Geometry check sheet. Reference: drawing and pictorial views, mm from the part's lowest x, y, z. A direction names the side the tool comes from. Round coordinates to 2 decimals unless told otherwise and drop trailing zeros. Write each loop counter-clockwise with the first axis right and the second up, starting at its lowest first coordinate (ties: lowest second). Pieces come first, ordered by that corner, then holes. Notation, with made-up numbers: M -23.5,47 L 4.5,47 A31 ccw 4.5,74 Z; hole C 75.25,85.5 d6. An arc over 180 degrees is marked long. One line per item, written item: value. Start each with the question number.
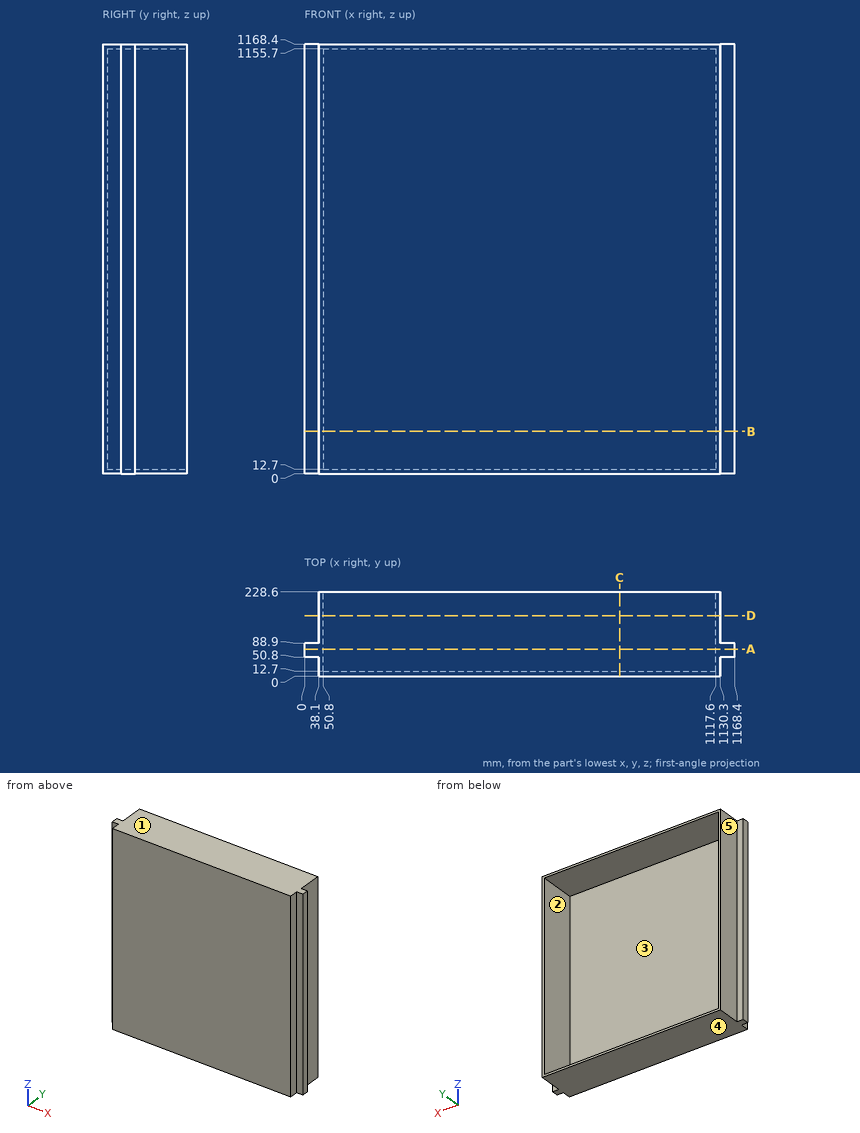
1) Access from +Z, -Z, +X, -X, +Y, -Y to the whole of each face (thin tool, end or side, straight path). Record for the marked faces 1 and 2.
2) Gauge pin test, flat ends, axial feed: pin 1 Ø19 at (x, z) = (1140.5, 494.5) entering from -Y; pin 2 Ø10 at (x, z) = (166, 423.5) entering from +Y; pin 3 Ø2 at (y, z) = (147.5, 708) entering from -X. Record the tip position at first contact, or that the pin passes through.
3) Cross-section at D-D (y = 164). Record the boundary of the cut face in (x, z), then the cut area to 3 significant figures.
4) Thickness scan on line 1 (Z direction, x = 68, y = 71); line 2 (X direction, y = 132, z = 960); line 3 (X direction, y = 84, z = 931.5). Record the ranges inside material, lowest first.
5) Mould release check, pull along X, two halves, no side actions. Record for the marked faces 3, 4 and 5: pulls with the +X half, pulls with the -X half, needs draft (parallel to the pull), parting line crosses it, or undercut.
6) Cross-section at A-A (y = 73). Record the boundary of the cut face in (x, z), then the cut area to 3 significant figures.
7) Cross-section at B-B (z = 115.5). Record the boundary of the cut face in (x, y), then the cut area to 3 significant figures.
8) Cross-section at C-C (x = 856). Record the boundary of the cut face in (y, z).
Results below:
1. face 1: +Z, +X, -X, +Y, -Y
1. face 2: +Y
2. pin 1: stops at y = 50.8
2. pin 2: stops at y = 12.7
2. pin 3: stops at x = 38.1
3. outline: M 38.1,0 L 1130.3,0 L 1130.3,1168.4 L 38.1,1168.4 Z; hole M 50.8,12.7 L 1117.6,12.7 L 1117.6,1155.7 L 50.8,1155.7 Z
3. area: 56,800 mm²
4. line 1: z = 0 to 12.7, 1155.7 to 1168.4
4. line 2: x = 38.1 to 50.8, 1117.6 to 1130.3
4. line 3: x = 0 to 50.8, 1117.6 to 1168.4
5. face 3: undercut
5. face 4: needs draft
5. face 5: pulls with the -X half
6. outline: M 0,0 L 1168.4,0 L 1168.4,1168.4 L 0,1168.4 Z; hole M 50.8,12.7 L 1117.6,12.7 L 1117.6,1155.7 L 50.8,1155.7 Z
6. area: 146,000 mm²
7. outline: M 0,50.8 L 38.1,50.8 L 38.1,0 L 1130.3,0 L 1130.3,50.8 L 1168.4,50.8 L 1168.4,88.9 L 1130.3,88.9 L 1130.3,228.6 L 1117.6,228.6 L 1117.6,12.7 L 50.8,12.7 L 50.8,228.6 L 38.1,228.6 L 38.1,88.9 L 0,88.9 Z
7. area: 22,300 mm²
8. outline: M 0,0 L 228.6,0 L 228.6,12.7 L 12.7,12.7 L 12.7,1155.7 L 228.6,1155.7 L 228.6,1168.4 L 0,1168.4 Z
